Print and shaded views of the part. All mm, measured from the part's lowest x, y and z. A direction names the side the tool comes from. Give positions to 0.01 mm unless a question says otherwise; leave off trailing zeros. Write each loop counter-clockwise with the first axis right and the second up, starting at its lowest first coordinate (ties: lowest second). Pieces come first, ordered by that corner, then holes. Notation, with made-up numbers: (46, 62) -> (51, 62) arc R19 cw to (51, 91) -> close; hole circle Ø5 at (-39.75, 68). An arc over 180 degrees is marked (long way). Put each result on its own line as item: value.
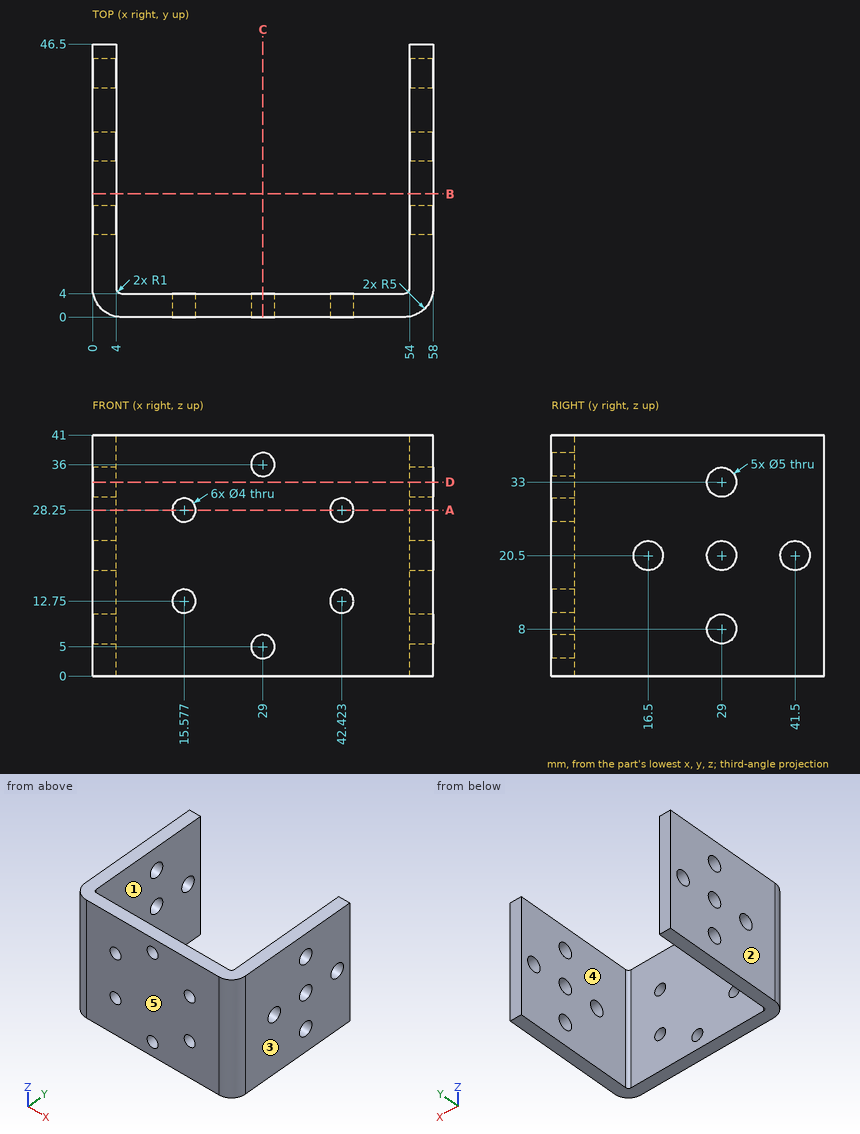
1) Tool access for the marked faces 1 and 2: list every direction of +Z, -Z, +X, -X, +Y, -Y with a clear straight run to the whole face (end or side of a thin tool).
Filled sheet:
face 1: +Z, -Z, +Y
face 2: +Z, -Z, -X, +Y, -Y
2) Wall check: L1, parallel to X at y = 26, z = 14; L2, parallel to Y at x = 21.5, z = 11.5; L3, parallel to Z at x = 55, y = 41. Give the ranges that are in metal, low to high.
Filled sheet:
L1: 0 to 4, 54 to 58
L2: 0 to 4
L3: 0 to 18.05, 22.95 to 41
3) Pull direction X, two halves, no side cores. Call the marked faces 3, 4 and 5: released by +X, released by -X, zero draft, split by the parting line, or undercut.
Filled sheet:
face 3: released by +X
face 4: undercut
face 5: zero draft
4) Slice it at B-B (y = 21). Write the cut outline in (x, z), plus the area to 3 significant figures.
Filled sheet:
outline: (0, 0) -> (4, 0) -> (4, 41) -> (0, 41) -> close; (54, 0) -> (58, 0) -> (58, 41) -> (54, 41) -> close
area: 328 mm2
5) Pin check, flat tip, straight feed: pin 1 (5 mm diameter, centred on x = 32.5, z = 36.5, fed in from +Y). Stop position of the tip, or through.
Filled sheet:
pin 1: y = 4
6) Slice it at C-C (x = 29). Write the cut outline in (y, z).
Filled sheet:
outline: (0, 0) -> (4, 0) -> (4, 3) -> (0, 3) -> close; (0, 7) -> (4, 7) -> (4, 34) -> (0, 34) -> close; (0, 38) -> (4, 38) -> (4, 41) -> (0, 41) -> close
7) Slice it at A-A (z = 28.25). Write the cut outline in (x, y).
Filled sheet:
outline: (0, 5) arc R5 ccw to (5, 0) -> (13.58, 0) -> (13.58, 4) -> (5, 4) arc R1 cw to (4, 5) -> (4, 46.5) -> (0, 46.5) -> close; (17.58, 0) -> (40.42, 0) -> (40.42, 4) -> (17.58, 4) -> close; (44.42, 0) -> (53, 0) arc R5 ccw to (58, 5) -> (58, 46.5) -> (54, 46.5) -> (54, 5) arc R1 cw to (53, 4) -> (44.42, 4) -> close
8) Slice it at D-D (z = 33). Write the cut outline in (x, y).
Filled sheet:
outline: (0, 5) arc R5 ccw to (5, 0) -> (53, 0) arc R5 ccw to (58, 5) -> (58, 26.5) -> (54, 26.5) -> (54, 5) arc R1 cw to (53, 4) -> (5, 4) arc R1 cw to (4, 5) -> (4, 26.5) -> (0, 26.5) -> close; (0, 31.5) -> (4, 31.5) -> (4, 46.5) -> (0, 46.5) -> close; (54, 31.5) -> (58, 31.5) -> (58, 46.5) -> (54, 46.5) -> close
